Check sheet for the drawn part. Datum: minimum x, y, z corner. Units: mm. A direction names the side the tool comes from. Coordinates: 2 decimals unless noted, no trailing zeros. Write each loop counter-clockwise with the first axis right and the second up, starting at its lowest first coordinate (ties: lowest second). Pieces come first, ordered by that corner, then holes. Notation, with made-up numbers: (69, 47) - (127, 47) arc R7 cw to (127, 53) - close; hole circle Ø4 at (44.5, 46.25). An arc over 180 degrees is marked (long way). Use one line per item in the form item = value. Start each with the question number.
1. Cross-section at C-C on y = 11. Record the boundary of the cut face in (x, z).
2. Cross-section at B-B on x = 2.7. Record the boundary of the cut face in (y, z), then the cut area to 3 significant figures.
3. Scan lines: line 1 along X through (y, z) = (9.4, 15); line 2 along Z through (x, y) = (2.7, 9.2); line 3 along Y through (x, z) = (10.75, 13). Record each from-to range of solid material in increasing order.
4. Draft check along Z on the marked faces 1, 2 and 3. Enter one of: +Z half, -Z half, draft (parallel to the pull), parting line (faces both ways), or undercut.
5. Go/stop test with flat-tipped pins: pin 1 Ø1.5 at (x, z) = (8, 6.5) entering from +Y; pin 2 Ø1 at (y, z) = (11, 15.5) entering from -X; pin 3 Ø6 at (x, z) = (21, 7.5) entering from -Y; pin 4 Ø9 at (x, z) = (16, 12.5) entering from +Y. Record where each tip stops, or that it passes through.
6. Cross-section at A-A on z = 15. Record the boundary of the cut face in (x, y), then the cut area to 3 significant figures.
7. Tool access check on the marked faces 4, 5, 6 and 7. Record the directions out of +Z, -Z, +X, -X, +Y, -Y that give a thin tool (end or side, any length) a straight path to the whole face; none if there is none.
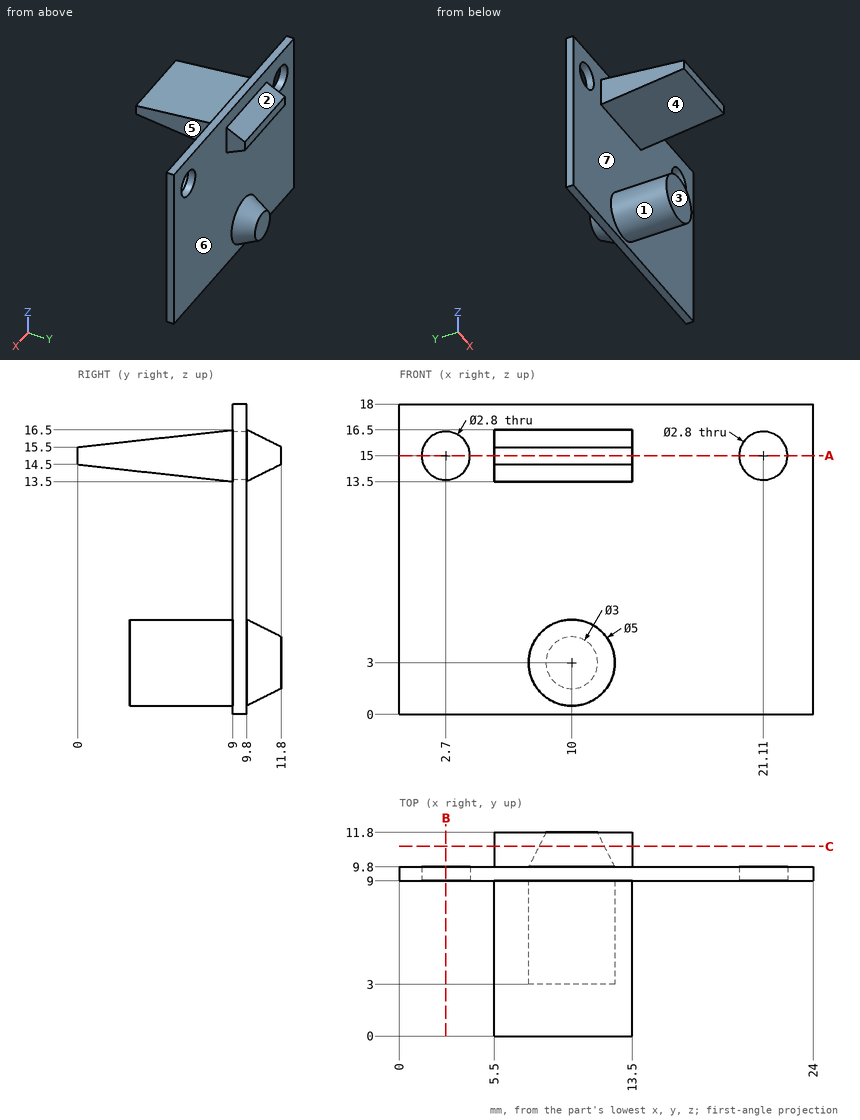
Final values:
q1.outline = (5.5, 14.1) - (13.5, 14.1) - (13.5, 15.9) - (5.5, 15.9) - close; circle Ø3.8 at (10, 3)
q2.outline = (9, 0) - (9.8, 0) - (9.8, 13.6) - (9, 13.6) - close; (9, 16.4) - (9.8, 16.4) - (9.8, 18) - (9, 18) - close
q2.area = 12.2 mm²
q3.line_1 = 0 to 1.3, 4.1 to 19.71, 22.51 to 24
q3.line_2 = 0 to 13.6, 16.4 to 18
q3.line_3 = 9 to 9.8
q4.face_1 = undercut
q4.face_2 = +Z half
q4.face_3 = draft
q5.pin_1 = 9.8
q5.pin_2 = 5.5
q5.pin_3 = 9
q5.pin_4 = 11.8
q6.outline = (0, 9) - (1.3, 9) - (1.3, 9.8) - (0, 9.8) - close; (4.1, 9) - (5.5, 9) - (5.5, 0) - (13.5, 0) - (13.5, 9) - (19.71, 9) - (19.71, 9.8) - (13.5, 9.8) - (13.5, 11.8) - (5.5, 11.8) - (5.5, 9.8) - (4.1, 9.8) - close; (22.51, 9) - (24, 9) - (24, 9.8) - (22.51, 9.8) - close
q6.area = 103 mm²
q7.face_4 = +X, -X, -Y
q7.face_5 = +Z, -Z, +X, -Y
q7.face_6 = +Y
q7.face_7 = -Y
